Could you check a few things on this model? Use its own coordinates, in mm. Face numbers are marked on the shaded views. Round coordinates to 2 decimals unless told otherwise and drop trailing zeros. Loops run counter-clockwise (first coordinate to the right, second up) from the corner with the lowest first, then second, coordinate; pieces in that order, holes last. Notation, with made-up numbers: (-28.75, 70) - (-21.75, 70) arc R19 cw to (-21.75, 77) - close; hole circle Ø5 at (54, 55.25). An arc over 180 degrees is marked (long way). Answer as CSV lines item,"result". Start each with the question number.
1) I'm going to push flat-ended pins straight in: pin 1 Ø0.7 at (x, z) = (3.5, 2) entering from +Y; pin 2 Ø1.5 at (x, z) = (-2, 3) entering from -Y; pin 3 Ø4 at (x, y) = (0, 0.5) entering from -Z. Where does each tip first touch, or does it pass through?
2) Suppose I cut it at B-B, the plane x = 0. Write out the boundary of the cut face in (y, z) (3 decimals).
3) We'd pull the mould along X, two halves only. Please class the marked faces 1, 2 and 3: pulls with the +X half, pulls with the -X half, needs draft (parallel to the pull), parting line crosses it, or undercut.
4) Suppose I cut it at C-C, the plane y = 4.75. Write out the boundary of the cut face in (x, z) (3 decimals), then the cut area to 3 significant figures.
5) Please list where these lines run through material, in increasing order: line 1 along X through (y, z) = (-3.5, 1.5) (3 decimals); line 2 along Z through (x, y) = (-2.5, 3.5); line 3 along X through (y, z) = (1.75, 2.5).
6) Suppose I cut it at A-A, the plane z = -2. Count the separate pieces of the cut face and the enclosed holes in it, then the cut area to 3 significant figures.
```python
from build123d import *

# Parameters (mm, degrees)
BASIC_SHAPE_DEPTH              = 5.46
SIDE_PROFILE1_DEPTH            = 9.155243712
SIDE_PROFILE1_DEPTH_BACK       = 9.155243712
SIDE_PROFILE2_DEPTH            = 9.155243712
SIDE_PROFILE2_DEPTH_BACK       = 9.155243712
LOCATION_MARK_DEPTH            = 0.8
SKETCH6_W                      = 0.25
SKETCH6_H                      = 1.39
PIN_RELIEF_DEPTH               = 11.390535357
REMAINING_PINS_COUNT           = 4
REMAINING_PINS_PITCH           = 2.54
REMAINING_PINS_COPY_1_SKETCH_W = 0.25
REMAINING_PINS_COPY_1_SKETCH_H = 1.39
REMAINING_PINS_COPY_2_SKETCH_W = 0.25
REMAINING_PINS_COPY_2_SKETCH_H = 1.39
REMAINING_PINS_COPY_3_SKETCH_W = 0.25
REMAINING_PINS_COPY_3_SKETCH_H = 1.39
REMAINING_PINS_COPY_4_DEPTH    = 11.390535357
REMAINING_PINS_COPY_5_DEPTH    = 11.390535357
REMAINING_PINS_COPY_6_DEPTH    = 11.390535357
PIN_SHAPE1_DEPTH               = 0.445
PIN_SHAPE2_DEPTH               = 0.445


with BuildPart() as part:
    # Sketch1 → Basic Shape (new, symmetric)
    with BuildSketch(Plane(origin=(0, 0, 0), x_dir=(1, 0, 0), z_dir=(0, 1, 0))):
        Polygon((-3.05, -0.51), (-3.3, -2.795), (-3.05, -5.08), (3.05, -5.08), (3.3, -2.795), (3.05, -0.51), align=None)
    extrude(amount=BASIC_SHAPE_DEPTH, both=True)

    # Sketch2 → Side Profile1 (cut, two sides: drawn at the far end of the back side and taken through both)
    with BuildSketch(Plane(origin=(0, 0, 0), x_dir=(0, 0, -1), z_dir=(1, 0, 0)).offset(-SIDE_PROFILE1_DEPTH_BACK)):
        Polygon((-5.08, 5.46), (-5.08, 5.21), (-2.795, 5.46), align=None)
        Polygon((-5.08, -5.46), (-2.795, -5.46), (-5.08, -5.21), align=None)
    extrude(amount=SIDE_PROFILE1_DEPTH + SIDE_PROFILE1_DEPTH_BACK, mode=Mode.SUBTRACT)

    # Sketch3 → Side Profile2 (cut, two sides: drawn at the far end of the back side and taken through both)
    with BuildSketch(Plane(origin=(0, 0, 0), x_dir=(0, 0, -1), z_dir=(1, 0, 0)).offset(-SIDE_PROFILE2_DEPTH_BACK)):
        Polygon((-2.795, 5.46), (-0.51, 5.46), (-0.51, 5.21), align=None)
        Polygon((-2.795, -5.46), (-0.51, -5.46), (-0.51, -5.21), align=None)
    extrude(amount=SIDE_PROFILE2_DEPTH + SIDE_PROFILE2_DEPTH_BACK, mode=Mode.SUBTRACT)

    # Sketch4 → Location Mark (cut)
    with BuildSketch(Plane(origin=(0, 0, 5.08), x_dir=(-1, 0, 0), z_dir=(0, 0, -1))):
        with BuildLine():
            Line((0.7, 5.563480235), (0.7, 4.063480235))
            ThreePointArc((0.7, 4.063480235), (0, 3.363480235), (-0.7, 4.063480235))
            Line((-0.7, 4.063480235), (-0.7, 5.563480235))
            Line((-0.7, 5.563480235), (0.7, 5.563480235))
        make_face()
    extrude(amount=LOCATION_MARK_DEPTH, mode=Mode.SUBTRACT)

    # First Pin: sweep along a path in Sketch5
    with BuildLine(Plane(origin=(0, -3.94, 0), x_dir=(1, 0, 0), z_dir=(0, 1, 0))) as first_pin_path:
        Line((0, -2.795), (3.31, -2.795))
        ThreePointArc((3.31, -2.795), (3.663553391, -2.648553391), (3.81, -2.295))
        Line((3.81, -2.295), (3.81, 3.5))
    # Sketch6 → First Pin (sweep)
    with BuildSketch(Plane(origin=(0, 0, 0), x_dir=(0, 0, -1), z_dir=(1, 0, 0))):
        with Locations((-2.795, -3.94)):
            Rectangle(SKETCH6_W, SKETCH6_H)
    first_pin = sweep(path=first_pin_path.line)

    # Sketch7 → Pin Relief (cut, through all)
    with BuildSketch(Plane(origin=(3.935, 0, 0), x_dir=(0, 0, -1), z_dir=(1, 0, 0))):
        Polygon((0, -4.19), (3.5, -4.19), (3.5, -4.635), (-0.51, -4.635), (0, -4.4125), align=None)
        Polygon((0, -3.69), (3.5, -3.69), (3.5, -3.245), (-0.51, -3.245), (0, -3.4675), align=None)
    pin_relief = extrude(amount=-PIN_RELIEF_DEPTH, mode=Mode.SUBTRACT)

    # Opp Pin: First Pin, Pin Relief across plane
    add(first_pin.mirror(Plane(origin=(0, 0, 0), x_dir=(0, 0, 1), z_dir=(1, 0, 0))))
    add(pin_relief.mirror(Plane(origin=(0, 0, 0), x_dir=(0, 0, 1), z_dir=(1, 0, 0))), mode=Mode.SUBTRACT)

    # Remaining Pins: First Pin, Pin Relief ×4
    with Locations(*[(0, i * REMAINING_PINS_PITCH, 0) for i in range(1, REMAINING_PINS_COUNT)]):
        add(first_pin)
        add(pin_relief, mode=Mode.SUBTRACT)

    # Remaining Pins copy 1: sweep along a path in Remaining Pins copy 1 path
    with BuildLine(Plane(origin=(0, -1.4, 0), x_dir=(-1, 0, 0), z_dir=(0, 1, 0))) as remaining_pins_copy_1_path:
        Line((0, 2.795), (3.31, 2.795))
        ThreePointArc((3.31, 2.795), (3.663553391, 2.648553391), (3.81, 2.295))
        Line((3.81, 2.295), (3.81, -3.5))
    # Remaining Pins copy 1 sketch → Remaining Pins copy 1 (sweep)
    with BuildSketch(Plane(origin=(0, 2.54, 0), x_dir=(0, 0, -1), z_dir=(-1, 0, 0))):
        with Locations((-2.795, 3.94)):
            Rectangle(REMAINING_PINS_COPY_1_SKETCH_W, REMAINING_PINS_COPY_1_SKETCH_H)
    sweep(path=remaining_pins_copy_1_path.line)

    # Remaining Pins copy 2: sweep along a path in Remaining Pins copy 2 path
    with BuildLine(Plane(origin=(0, 1.14, 0), x_dir=(-1, 0, 0), z_dir=(0, 1, 0))) as remaining_pins_copy_2_path:
        Line((0, 2.795), (3.31, 2.795))
        ThreePointArc((3.31, 2.795), (3.663553391, 2.648553391), (3.81, 2.295))
        Line((3.81, 2.295), (3.81, -3.5))
    # Remaining Pins copy 2 sketch → Remaining Pins copy 2 (sweep)
    with BuildSketch(Plane(origin=(0, 5.08, 0), x_dir=(0, 0, -1), z_dir=(-1, 0, 0))):
        with Locations((-2.795, 3.94)):
            Rectangle(REMAINING_PINS_COPY_2_SKETCH_W, REMAINING_PINS_COPY_2_SKETCH_H)
    sweep(path=remaining_pins_copy_2_path.line)

    # Remaining Pins copy 3: sweep along a path in Remaining Pins copy 3 path
    with BuildLine(Plane(origin=(0, 3.68, 0), x_dir=(-1, 0, 0), z_dir=(0, 1, 0))) as remaining_pins_copy_3_path:
        Line((0, 2.795), (3.31, 2.795))
        ThreePointArc((3.31, 2.795), (3.663553391, 2.648553391), (3.81, 2.295))
        Line((3.81, 2.295), (3.81, -3.5))
    # Remaining Pins copy 3 sketch → Remaining Pins copy 3 (sweep)
    with BuildSketch(Plane(origin=(0, 7.62, 0), x_dir=(0, 0, -1), z_dir=(-1, 0, 0))):
        with Locations((-2.795, 3.94)):
            Rectangle(REMAINING_PINS_COPY_3_SKETCH_W, REMAINING_PINS_COPY_3_SKETCH_H)
    sweep(path=remaining_pins_copy_3_path.line)

    # Remaining Pins copy 4 sketch → Remaining Pins copy 4 (cut, through all)
    with BuildSketch(Plane(origin=(-3.935, 2.54, 0), x_dir=(0, 0, -1), z_dir=(-1, 0, 0))):
        Polygon((0, 4.19), (3.5, 4.19), (3.5, 4.635), (-0.51, 4.635), (0, 4.4125), align=None)
        Polygon((0, 3.69), (3.5, 3.69), (3.5, 3.245), (-0.51, 3.245), (0, 3.4675), align=None)
    extrude(amount=-REMAINING_PINS_COPY_4_DEPTH, mode=Mode.SUBTRACT)

    # Remaining Pins copy 5 sketch → Remaining Pins copy 5 (cut, through all)
    with BuildSketch(Plane(origin=(-3.935, 5.08, 0), x_dir=(0, 0, -1), z_dir=(-1, 0, 0))):
        Polygon((0, 4.19), (3.5, 4.19), (3.5, 4.635), (-0.51, 4.635), (0, 4.4125), align=None)
        Polygon((0, 3.69), (3.5, 3.69), (3.5, 3.245), (-0.51, 3.245), (0, 3.4675), align=None)
    extrude(amount=-REMAINING_PINS_COPY_5_DEPTH, mode=Mode.SUBTRACT)

    # Remaining Pins copy 6 sketch → Remaining Pins copy 6 (cut, through all)
    with BuildSketch(Plane(origin=(-3.935, 7.62, 0), x_dir=(0, 0, -1), z_dir=(-1, 0, 0))):
        Polygon((0, 4.19), (3.5, 4.19), (3.5, 4.635), (-0.51, 4.635), (0, 4.4125), align=None)
        Polygon((0, 3.69), (3.5, 3.69), (3.5, 3.245), (-0.51, 3.245), (0, 3.4675), align=None)
    extrude(amount=-REMAINING_PINS_COPY_6_DEPTH, mode=Mode.SUBTRACT)

    # Sketch9 → Pin Shape1 (cut)
    with BuildSketch(Plane.XZ.offset(4.635)):
        with BuildLine():
            Line((3.935, 0), (3.685, 0))
            Line((3.685, 0), (3.685, 2.295))
            ThreePointArc((3.685, 2.295), (3.575165043, 2.560165043), (3.31, 2.67))
            Line((3.31, 2.67), (3.286323851, 2.67))
            Line((3.286323851, 2.67), (3.3, 2.795))
            Line((3.3, 2.795), (3.286323851, 2.92))
            Line((3.286323851, 2.92), (3.31, 2.92))
            ThreePointArc((3.31, 2.92), (3.751941738, 2.736941738), (3.935, 2.295))
            Line((3.935, 2.295), (3.935, 0))
        make_face()
        with BuildLine():
            Line((-3.685, 0), (-3.935, 0))
            Line((-3.935, 0), (-3.935, 2.295))
            ThreePointArc((-3.935, 2.295), (-3.751941738, 2.736941738), (-3.31, 2.92))
            Line((-3.31, 2.92), (-3.286323851, 2.92))
            Line((-3.286323851, 2.92), (-3.3, 2.795))
            Line((-3.3, 2.795), (-3.286323851, 2.67))
            Line((-3.286323851, 2.67), (-3.31, 2.67))
            ThreePointArc((-3.31, 2.67), (-3.575165043, 2.560165043), (-3.685, 2.295))
            Line((-3.685, 2.295), (-3.685, 0))
        make_face()
    extrude(amount=-PIN_SHAPE1_DEPTH, mode=Mode.SUBTRACT)

    # Sketch10 → Pin Shape2 (cut)
    with BuildSketch(Plane(origin=(0, 4.375, 0), x_dir=(-1, 0, 0), z_dir=(0, 1, 0))):
        with BuildLine():
            Line((3.685, 0), (3.935, 0))
            Line((3.935, 0), (3.935, 2.295))
            ThreePointArc((3.935, 2.295), (3.751941738, 2.736941738), (3.31, 2.92))
            Line((3.31, 2.92), (3.286323851, 2.92))
            Line((3.286323851, 2.92), (3.3, 2.795))
            Line((3.3, 2.795), (3.286323851, 2.67))
            Line((3.286323851, 2.67), (3.31, 2.67))
            ThreePointArc((3.31, 2.67), (3.575165043, 2.560165043), (3.685, 2.295))
            Line((3.685, 2.295), (3.685, 0))
        make_face()
        with BuildLine():
            Line((-3.685, 0), (-3.935, 0))
            Line((-3.935, 0), (-3.935, 2.295))
            ThreePointArc((-3.935, 2.295), (-3.751941738, 2.736941738), (-3.31, 2.92))
            Line((-3.31, 2.92), (-3.286323851, 2.92))
            Line((-3.286323851, 2.92), (-3.3, 2.795))
            Line((-3.3, 2.795), (-3.286323851, 2.67))
            Line((-3.286323851, 2.67), (-3.31, 2.67))
            ThreePointArc((-3.31, 2.67), (-3.575165043, 2.560165043), (-3.685, 2.295))
            Line((-3.685, 2.295), (-3.685, 0))
        make_face()
    extrude(amount=-PIN_SHAPE2_DEPTH, mode=Mode.SUBTRACT)


solid = part.part
```
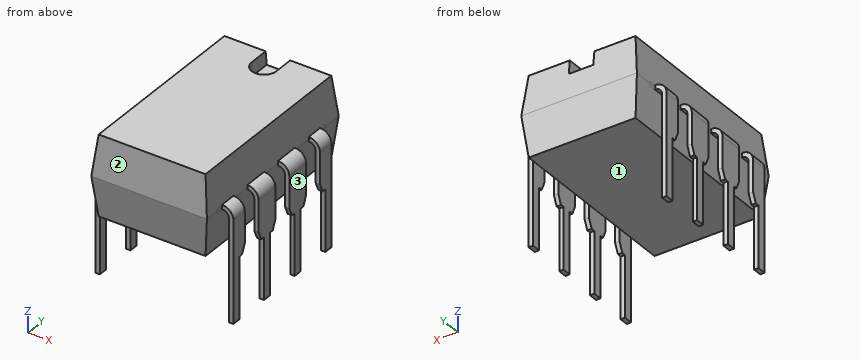
Filled sheet:
1,pin 1,"y = 5.4"
1,pin 2,"y = -5.46"
1,pin 3,"z = 0.51"
2,outline,"(-5.46, 2.795) - (-5.21, 0.51) - (5.21, 0.51) - (5.46, 2.795) - (5.298, 4.28) - (3.363, 4.28) - (3.363, 5.08) - (-5.21, 5.08) - close"
3,face 1,"undercut"
3,face 2,"needs draft"
3,face 3,"pulls with the +X half"
4,outline,"(-3.3, 2.795) - (-3.05, 0.51) - (3.05, 0.51) - (3.3, 2.795) - (3.05, 5.08) - (0.7, 5.08) - (0.7, 4.28) - (-0.7, 4.28) - (-0.7, 5.08) - (-3.05, 5.08) - close"
4,area,"27.9 mm²"
5,line 1,"-3.935 to -3.685, -3.158 to 3.158, 3.685 to 3.935"
5,line 2,"0.51 to 5.08"
5,line 3,"-3.9 to -3.62, -3.27 to 3.27, 3.62 to 3.9"
6,separate pieces,"8"
6,enclosed holes,"0"
6,area,"1.00 mm²"
